Geometry: final body of the model. Coordinates: model frame, mm. Face numbers are marked on the shaded views. Round coordinates to 2 decimals unless told otherwise and drop trailing zeros. Loops run counter-clockwise (first coordinate to the right, second up) from the corner with the lowest first, then second, coordinate; pieces in that order, holes last. Notation, with made-up numbers: (-4, 0) - (10, 0) arc R26 ccw to (10, 22) - close; hole circle Ø2 at (82, 18.25). An arc over 180 degrees is marked (long way). Answer in a Markdown table with one row per item. Add a question column.
from build123d import *

# Parameters (mm, degrees)
F0_R     = 83.5
F1_DEPTH = 231
F2_R     = 20
F3_T     = -2
F5_DEPTH = 84.5000001
F6_R     = 55
F7_DEPTH = 25


with BuildPart() as f1:
    # F0 (on Top) → F1 (new body)
    with BuildSketch(Plane.XY):
        Circle(F0_R)
    extrude(amount=F1_DEPTH)

    # F2
    f2_edges = [f1.edges().sort_by_distance(p)[0] for p in [
        (-83.5, 0, 231),
    ]]
    fillet(f2_edges, radius=F2_R)

    # F3
    f3_openings = [f1.faces().sort_by_distance(p)[0] for p in [
        (0, 0, 0),
    ]]
    offset(amount=F3_T, openings=f3_openings)

    # F4 (on Front) → F5 (cut, up to face)
    with BuildSketch(Plane.XZ):
        with BuildLine():
            Line((-15, 20), (15, 20))
            ThreePointArc((15, 20), (22.0710678119, 22.9289321881), (25, 30))
            Line((25, 30), (25, 160))
            ThreePointArc((25, 160), (22.0710678119, 167.0710678119), (15, 170))
            Line((15, 170), (-15, 170))
            ThreePointArc((-15, 170), (-22.0710678119, 167.0710678119), (-25, 160))
            Line((-25, 160), (-25, 30))
            ThreePointArc((-25, 30), (-22.0710678119, 22.9289321881), (-15, 20))
        make_face()
    extrude(amount=F5_DEPTH, mode=Mode.SUBTRACT)

    # F6 (on face) → F7 (cut)
    with BuildSketch(Plane.XY.offset(231)):
        Circle(F6_R)
    extrude(amount=-F7_DEPTH, mode=Mode.SUBTRACT)


solid = f1.part
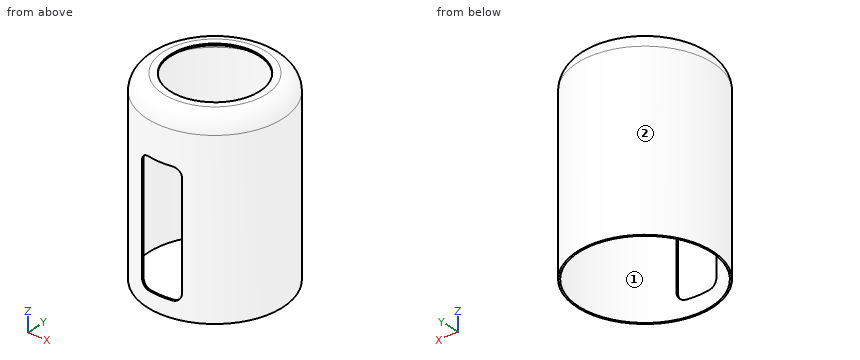
1) Section B-B, the plane x = 0. Return the cut outline in (y, z), and give its area (3 significant figures).
2) Material intervals for line 1 along X through (y, z) = (-47.5, 94.5); line 2 along Z through (x, y) = (-29, 54); line 3 along X through (y, z) = (72, 41), sorted ascending. Write a range as from..to.
3) Section A-A, the plane y = 0. Return the cut outline in (x, z), and give its area (3 significant figures).
4) Pull-direction query (Y, two-part tool) for the marked faces 1 and 2; classes: pulls with the +Y half, pulls with the -Y half, needs draft (parallel to the pull), parting line crosses it, or undercut.
5) Section D-D, the plane x = 22. Give the number of separate pieces and of enclosed holes in the cut face, and give its area (3 significant figures).
6) Section C-C, the plane z = 35.5. Return the cut outline in (x, y), and give its area (3 significant figures).
7) Contact query for flat-ended pins moving along their axis: pin 1 Ø3.5 at (x, y) = (-1, -82) entering from +Z; pin 2 Ø4 at (x, z) = (43.5, 69.5) entering from +Y; pin 3 Ø3 at (x, y) = (4, 59.5) entering from -Z; pin 4 Ø3.5 at (x, y) = (-0.5, -82.5) entering from -Z. Output: stop coordinate, or through.
Evaluation:
| question | item | result |
|---|---|---|
| 1 | outline | (-83.5, 0) - (-81.5, 0) - (-81.5, 20) - (-83.5, 20) - close; (-83.5, 170) - (-81.5, 170) - (-81.5, 211) arc R18 cw to (-63.5, 229) - (-55, 229) - (-55, 231) - (-63.5, 231) arc R20 ccw to (-83.5, 211) - close; (55, 229) - (63.5, 229) arc R18 cw to (81.5, 211) - (81.5, 0) - (83.5, 0) - (83.5, 211) arc R20 ccw to (63.5, 231) - (55, 231) - close |
| 1 | area | 697 mm² |
| 2 | line 1 | x = -68.67..-66.23, 66.23..68.67 |
| 2 | line 2 | z = 229..231 |
| 2 | line 3 | x = -42.29..-38.19, 38.19..42.29 |
| 3 | outline | (-83.5, 0) - (-81.5, 0) - (-81.5, 211) arc R18 cw to (-63.5, 229) - (-55, 229) - (-55, 231) - (-63.5, 231) arc R20 ccw to (-83.5, 211) - close; (55, 229) - (63.5, 229) arc R18 cw to (81.5, 211) - (81.5, 0) - (83.5, 0) - (83.5, 211) arc R20 ccw to (63.5, 231) - (55, 231) - close |
| 3 | area | 997 mm² |
| 4 | face 1 | undercut |
| 4 | face 2 | parting line crosses it |
| 5 | separate pieces | 3 |
| 5 | enclosed holes | 0 |
| 5 | area | 738 mm² |
| 6 | outline | (-25, -79.67) - (-25, -77.57) arc R81.5 cw (long way) to (25, -77.57) - (25, -79.67) arc R83.5 ccw (long way) to start |
| 6 | area | 935 mm² |
| 7 | pin 1 | stops at z = 221.92 |
| 7 | pin 2 | stops at y = 72.46 |
| 7 | pin 3 | stops at z = 229 |
| 7 | pin 4 | stops at z = 0 |
